from build123d import *

# Parameters (mm, degrees)
ESQUISSE2_R        = 2.75
BOSS_EXTRU_1_DEPTH = 32
ESQUISSE3_W        = 32
ESQUISSE3_H        = 16
ESQUISSE3_R        = 2.75
BOSS_EXTRU_2_DEPTH = 5


with BuildPart() as part:
    # Esquisse2 → Boss.-Extru.1 (new body)
    with BuildSketch(Plane.XY):
        with BuildLine():
            Line((-5.48727754, 19.978225401), (17.51272246, 19.978225401))
            Line((17.51272246, 19.978225401), (17.51272246, -28.021774599))
            Line((17.51272246, -28.021774599), (-5.48727754, -28.021774599))
            ThreePointArc((-5.48727754, -28.021774599), (-10.604983007, -27.469782846), (-15.48727754, -25.839198829))
            Line((-15.48727754, -25.839198829), (-15.48727754, -14.521774599))
            ThreePointArc((-15.48727754, -14.521774599), (9.01272246, -4.021774599), (-15.48727754, 6.478225401))
            Line((-15.48727754, 6.478225401), (-15.48727754, 17.79564963))
            ThreePointArc((-15.48727754, 17.79564963), (-10.604983007, 19.426233648), (-5.48727754, 19.978225401))
        make_face()
        with Locations((-5.48727754, 14.978225401)):
            Circle(ESQUISSE2_R, mode=Mode.SUBTRACT)
        with Locations((-5.48727754, -23.021774599)):
            Circle(ESQUISSE2_R, mode=Mode.SUBTRACT)
    extrude(amount=BOSS_EXTRU_1_DEPTH)

    # Esquisse3 → Boss.-Extru.2 (add)
    # profile 1 of 2: a face of its own
    with BuildSketch(Plane(origin=(17.51272246, 0, 0), x_dir=(0, 0, -1), z_dir=(1, 0, 0))):
        with Locations((-16, 27.978225401)):
            Rectangle(ESQUISSE3_W, ESQUISSE3_H)
        with Locations(Location((-16, 25.978225401, 0), (0, 0, 90))):
            Circle(ESQUISSE3_R, mode=Mode.SUBTRACT)
    # profile 2 of 2: a face of its own
    with BuildSketch(Plane(origin=(17.51272246, 0, 0), x_dir=(0, 0, -1), z_dir=(1, 0, 0))):
        with Locations((-16, -36.021774599)):
            Rectangle(ESQUISSE3_W, ESQUISSE3_H)
        with Locations(Location((-16, -34.021774599, 0), (0, 0, 90))):
            Circle(ESQUISSE3_R, mode=Mode.SUBTRACT)
    extrude(amount=-BOSS_EXTRU_2_DEPTH)


solid = part.part
The model under review builds one solid part; all positions refer to its coordinate system, in mm. A direction names the side the tool comes from. Give positions to 0.01 mm unless a question says otherwise; leave off trailing zeros. Loops run counter-clockwise (first coordinate to the right, second up) from the corner with the lowest first, then second, coordinate; pieces in that order, holes last. Notation, with made-up numbers: (10.5, 19) -> (26.5, 19) arc R23 ccw to (26.5, 54) -> close; hole circle Ø9 at (77.5, 12.25). An arc over 180 degrees is marked (long way). Answer as a JSON object with one key per item and string values. Group by question number.
Q1. Tool access review of faces 4 (the flat face through (12.513, -38, 16)), 5 (the cylindrical face through (9.005, -4.495, 15.776)), 6 (the flat face through (12.513, 30, 16)): name each direction out of +Z, -Z, +X, -X, +Y, -Y from which nothing blocks a thin tool from reaching the whole face with its end or side.
Q2. Insertion check: pin 1 (2 mm diameter, centred on x = 9, z = 8.5, fed in from -Y); pin 2 (14.5 mm diameter, centred on x = -0.5, z = 10.5, fed in from +Y); pin 3 (8 mm diameter, centred on y = -35.5, z = 11, fed in from -X). Each pin has a flat end and moves straight along its axis. Give the tip position at first contact, or say it passes through.
Q3. Draft analysis for pull direction X (two halves, no side actions). For faces 1 (the flat face through (4, -28.022, 16)), 2 (the flat face through (-15.487, 12, 16)), 3 (the cylindrical face through (-6.083, 12.294, 15.776)), state which applies: pulls with the +X half, pulls with the -X half, needs draft (parallel to the pull), parting line crosses it, or undercut.
Q4. Take a section at B-B (x = 3). Write out the cut boundary in (y, z).
Q5. Take a section at D-D (z = 30). Write out the cut boundary in (x, y).
Q6. Wall thickness on line 1 along Y through (x, z) = (-4, 28); line 2 along Y through (x, z) = (1, 5.5); line 3 along X through (y, z) = (-29.5, 5.5): over which ranges is each line inside the solid? List them lowest first.
Q7. Take a section at A-A (z = 16). Write out the cut boundary in (x, y).
Q8. Take a section at C-C (y = -33.5). Write out the cut boundary in (x, z).
Answer below:
{
 "1": {"face 4": "+Z, -Z, -X, -Y", "face 5": "+Z, -Z", "face 6": "+Z, -Z, -X, +Y"},
 "2": {"pin 1": "stops at y = -28.02", "pin 2": "stops at y = 19.98", "pin 3": "stops at x = 12.51"},
 "3": {"face 1": "needs draft", "face 2": "pulls with the -X half", "face 3": "undercut"},
 "4": {"outline": "(-28.02, 0) -> (-15.78, 0) -> (-15.78, 32) -> (-28.02, 32) -> close; (7.73, 0) -> (19.98, 0) -> (19.98, 32) -> (7.73, 32) -> close"},
 "5": {"outline": "(-15.49, -25.84) arc R24 ccw to (-5.49, -28.02) -> (12.51, -28.02) -> (12.51, -44.02) -> (17.51, -44.02) -> (17.51, 35.98) -> (12.51, 35.98) -> (12.51, 19.98) -> (-5.49, 19.98) arc R24 ccw to (-15.49, 17.8) -> (-15.49, 6.48) arc R14.5 cw (long way) to (-15.49, -14.52) -> close; hole circle Ø5.5 at (-5.49, -23.02); hole circle Ø5.5 at (-5.49, 14.98)"},
 "6": {"line 1": "y = -28.02 to -25.33, -20.71 to -18.45, 10.4 to 12.67, 17.29 to 19.98", "line 2": "y = -28.02 to -16.99, 8.95 to 19.98", "line 3": "x = 12.51 to 17.51"},
 "7": {"outline": "(-15.49, -25.84) arc R24 ccw to (-5.49, -28.02) -> (12.51, -28.02) -> (12.51, -31.27) -> (17.51, -31.27) -> (17.51, 23.23) -> (12.51, 23.23) -> (12.51, 19.98) -> (-5.49, 19.98) arc R24 ccw to (-15.49, 17.8) -> (-15.49, 6.48) arc R14.5 cw (long way) to (-15.49, -14.52) -> close; (12.51, -44.02) -> (17.51, -44.02) -> (17.51, -36.77) -> (12.51, -36.77) -> close; (12.51, 28.73) -> (17.51, 28.73) -> (17.51, 35.98) -> (12.51, 35.98) -> close; hole circle Ø5.5 at (-5.49, -23.02); hole circle Ø5.5 at (-5.49, 14.98)"},
 "8": {"outline": "(12.51, 0) -> (17.51, 0) -> (17.51, 13.3) -> (12.51, 13.3) -> close; (12.51, 18.7) -> (17.51, 18.7) -> (17.51, 32) -> (12.51, 32) -> close"}
}
